```python
from build123d import *

# Parameters (mm, degrees)
SKETCH_1_W          = 150
SKETCH_1_H          = 94
SKETCH_1_R          = 2.025
SKETCH_1_W_2        = 80
SKETCH_1_H_2        = 84
EXTRUDE_1_DEPTH     = 3
CHAMFER_1_SIZE      = 15
FILLET_1_R          = 10
SKETCH_2_W          = 14.5
SKETCH_2_H          = 82
CUT_EXTRUDE_1_DEPTH = 10
FILLET_2_R          = 2
SKETCH_3_R          = 1.525
CUT_EXTRUDE_2_DEPTH = 10


with BuildPart() as part:
    # 草图1 → 凸台-拉伸1 (new body)
    with BuildSketch(Plane.XY):
        with Locations((0, -2)):
            Rectangle(SKETCH_1_W, SKETCH_1_H)
        with Locations((-47.5, 0)):
            Circle(SKETCH_1_R, mode=Mode.SUBTRACT)
        with Locations((-47.5, 17)):
            Circle(SKETCH_1_R, mode=Mode.SUBTRACT)
        with Locations((-47.5, -25)):
            Circle(SKETCH_1_R, mode=Mode.SUBTRACT)
        with Locations((47.5, -25)):
            Circle(SKETCH_1_R, mode=Mode.SUBTRACT)
        with Locations((47.5, 17)):
            Circle(SKETCH_1_R, mode=Mode.SUBTRACT)
        with Locations((47.5, 0)):
            Circle(SKETCH_1_R, mode=Mode.SUBTRACT)
        with Locations((0, -2)):
            Rectangle(SKETCH_1_W_2, SKETCH_1_H_2, mode=Mode.SUBTRACT)
    extrude(amount=EXTRUDE_1_DEPTH)

    # 倒角1
    chamfer_1_edges = [part.edges().sort_by_distance(p)[0] for p in [
        (40, -44, 1.5),
        (40, 40, 1.5),
        (-40, 40, 1.5),
        (-40, -44, 1.5),
    ]]
    chamfer(chamfer_1_edges, length=CHAMFER_1_SIZE)

    # 圆角1
    fillet_1_edges = [part.edges().sort_by_distance(p)[0] for p in [
        (-25, -44, 1.5),
        (25, -44, 1.5),
        (40, 25, 1.5),
        (40, -29, 1.5),
        (-25, 40, 1.5),
        (25, 40, 1.5),
        (-40, -29, 1.5),
        (-40, 25, 1.5),
    ]]
    fillet(fillet_1_edges, radius=FILLET_1_R)

    # 草图2 → 切除-拉伸1 (cut)
    with BuildSketch(Plane.XY.offset(3)):
        with Locations((-61.75, -2)):
            Rectangle(SKETCH_2_W, SKETCH_2_H)
        with Locations((61.75, -2)):
            Rectangle(SKETCH_2_W, SKETCH_2_H)
    extrude(amount=-CUT_EXTRUDE_1_DEPTH, mode=Mode.SUBTRACT)

    # 圆角2
    fillet_2_edges = [part.edges().sort_by_distance(p)[0] for p in [
        (-69, -43, 1.5),
        (-69, 39, 1.5),
        (-54.5, 39, 1.5),
        (-54.5, -43, 1.5),
        (69, 39, 1.5),
        (69, -43, 1.5),
        (54.5, -43, 1.5),
        (54.5, 39, 1.5),
        (-75, 45, 1.5),
        (75, 45, 1.5),
        (75, -49, 1.5),
        (-75, -49, 1.5),
    ]]
    fillet(fillet_2_edges, radius=FILLET_2_R)

    # 草图3 → 切除-拉伸2 (cut)
    with BuildSketch(Plane.XY.offset(3)):
        with Locations((72, -9)):
            Circle(SKETCH_3_R)
        with Locations((72, -29)):
            Circle(SKETCH_3_R)
        with Locations((-72, -29)):
            Circle(SKETCH_3_R)
        with Locations((-72, -9)):
            Circle(SKETCH_3_R)
    extrude(amount=-CUT_EXTRUDE_2_DEPTH, mode=Mode.SUBTRACT)


solid = part.part
```
For this review, take the finished solid that the model builds, in its own axes (mm). A direction names the side the tool comes from. Coordinates: 2 decimals unless noted, no trailing zeros. Write each loop counter-clockwise with the first axis right and the second up, starting at its lowest first coordinate (ties: lowest second). Pieces come first, ordered by that corner, then holes. Notation, with made-up numbers: (81.5, 0) - (120.5, 0) arc R15 cw to (120.5, 6) - close; hole circle Ø8 at (-26, -40). An arc over 180 degrees is marked (long way). Answer in a Markdown table with one row per item. Add a question column.
Q1. We need section C-C, the plane y = -9. State the section outline as (x, z) points (3 decimals), and give its area (3 significant figures).
Q2. For P1, Ø6.5, axis at x = 47.5, y = 0, coming from the -Z side, flat-tipped, find the tip position at first contact; note if it passes through.
Q3. Draft analysis for pull direction X (two halves, no side actions). For faces 1 (the flat face through (-33, -36, 1)), 2 (the flat face through (-1, 45, 1)), 3 (the flat face through (32, 33, 1)), 4 (the flat face through (75, -3, 1)), state which applies: +X half, -X half, draft (parallel to the pull), parting line (faces both ways), or undercut.
Q4. We need section B-B, the plane x = -19. State the section outline as (y, z) points, and give its area (3 significant figures).
Q5. Tool access review of faces 5 (the flat face through (-1, -49, 1)), 6 (the flat face through (69, -3, 2)): name each direction out of +Z, -Z, +X, -X, +Y, -Y from which nothing blocks a thin tool from reaching the whole face with its end or side.
Q6. We need section A-A, the plane y = 30.5. State the section outline as (x, z) points, and give its area (3 significant figures).
Q7. For probe 1 along Y at (x, z) = (-47.5, 1.8) (3 decimals); probe 2 along X at (y, z) = (7, 2.2); probe 3 along Y at (x, z) = (72, 1.5) (3 decimals), list the stretches that pass through material, from the lowest coordinate up.
Q8. We need section D-D, the plane x = 47.5. State the section outline as (y, z) points (3 decimals), and give its area (3 significant figures).
Answer list:
| question | item | result |
|---|---|---|
| 1 | outline | (-75, 0) - (-73.525, 0) - (-73.525, 3) - (-75, 3) - close; (-70.475, 0) - (-69, 0) - (-69, 3) - (-70.475, 3) - close; (-54.5, 0) - (-40, 0) - (-40, 3) - (-54.5, 3) - close; (40, 0) - (54.5, 0) - (54.5, 3) - (40, 3) - close; (69, 0) - (70.475, 0) - (70.475, 3) - (69, 3) - close; (73.525, 0) - (75, 0) - (75, 3) - (73.525, 3) - close |
| 1 | area | 105 mm2 |
| 2 | P1 | stops at z = 0 |
| 3 | face 1 | undercut |
| 3 | face 2 | draft |
| 3 | face 3 | undercut |
| 3 | face 4 | +X half |
| 4 | outline | (-49, 0) - (-44, 0) - (-44, 3) - (-49, 3) - close; (40, 0) - (45, 0) - (45, 3) - (40, 3) - close |
| 4 | area | 30.0 mm2 |
| 5 | face 5 | +Z, -Z, +X, -X, -Y |
| 5 | face 6 | +Z, -Z |
| 6 | outline | (-75, 0) - (-69, 0) - (-69, 3) - (-75, 3) - close; (-54.5, 0) - (-34.5, 0) - (-34.5, 3) - (-54.5, 3) - close; (34.5, 0) - (54.5, 0) - (54.5, 3) - (34.5, 3) - close; (69, 0) - (75, 0) - (75, 3) - (69, 3) - close |
| 6 | area | 156 mm2 |
| 7 | probe 1 | y = -49 to -27.025, -22.975 to -2.025, 2.025 to 14.975, 19.025 to 45 |
| 7 | probe 2 | x = -75 to -69, -54.5 to -40, 40 to 54.5, 69 to 75 |
| 7 | probe 3 | y = -49 to -30.525, -27.475 to -10.525, -7.475 to 45 |
| 8 | outline | (-49, 0) - (-27.025, 0) - (-27.025, 3) - (-49, 3) - close; (-22.975, 0) - (-2.025, 0) - (-2.025, 3) - (-22.975, 3) - close; (2.025, 0) - (14.975, 0) - (14.975, 3) - (2.025, 3) - close; (19.025, 0) - (45, 0) - (45, 3) - (19.025, 3) - close |
| 8 | area | 246 mm2 |
